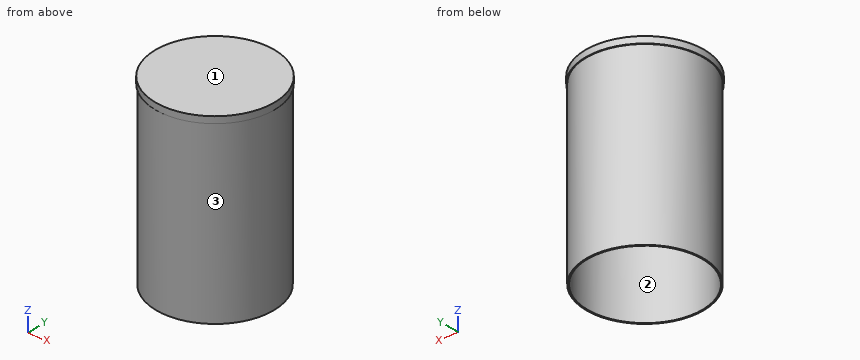
from build123d import *

# Parameters (mm, degrees)
CYLINDER_R      = 4.1
CYLINDER_DEPTH  = 3.1
SKETCH005_R     = 4.56
PAD002_DEPTH    = 0.5
SKETCH006_R     = 4.5
PAD003_DEPTH    = 13.5
SKETCH007_R     = 4.4
POCKET003_DEPTH = 13.5


with BuildPart() as part:
    # Cylinder → Cylinder (new body)
    with BuildSketch(Plane(origin=(-8, 0, 15.25), x_dir=(1, 0, 0), z_dir=(0, 0, 1))):
        Circle(CYLINDER_R)
    extrude(amount=CYLINDER_DEPTH)

    # Sketch005 → Pad002 (new body)
    with BuildSketch(Plane(origin=(-8, 0, 18.35), x_dir=(1, 0, 0), z_dir=(0, 0, 1))):
        Circle(SKETCH005_R)
    extrude(amount=PAD002_DEPTH)

    # Sketch006 → Pad003 (new body)
    with BuildSketch(Plane(origin=(-8, 0, 18.35), x_dir=(1, 0, 0), z_dir=(0, 0, -1))):
        Circle(SKETCH006_R)
    extrude(amount=PAD003_DEPTH)

    # Sketch007 → Pocket003 (cut)
    with BuildSketch(Plane(origin=(-8, 0, 4.85), x_dir=(1, 0, 0), z_dir=(0, 0, -1))):
        Circle(SKETCH007_R)
    extrude(amount=-POCKET003_DEPTH, mode=Mode.SUBTRACT)


solid = part.part
Could you check a few things on this model? Use its own coordinates, in mm. Face numbers are marked on the shaded views. Give positions to 0.01 mm unless a question says otherwise; leave off trailing zeros. Order: outer loops, then holes, each group sorted by start corner. A loop starts at its lowest first (then second) coordinate and runs counter-clockwise, first axis right, second up. Notation, with made-up numbers: (23.5, 0) -> (56.5, 0) arc R24 ccw to (56.5, 31) -> close; hole circle Ø4 at (13.5, 16). An arc over 180 degrees is marked (long way). Answer in a Markdown table with one row per item. Add a question column.
Item 1: I'm going to push flat-ended pins straight in: P1, Ø3, axis at y = -2.5, z = 8, coming from the -X side; P2, Ø2, axis at x = -4.5, z = 17, coming from the -Y side; P3, Ø2.5, axis at x = -9, y = 0, coming from the -Z side. Where does each tip first touch, or does it pass through?
Item 2: Imagine slicing it at A-A (x = -8.5). List the corners of the cut face in (y, z) for me.
Item 3: We'd pull the mould along Y, two halves only. Please class the marked faces 1, 2 and 3: pulls with the +Y half, pulls with the -Y half, needs draft (parallel to the pull), parting line crosses it, or undercut.
Item 4: Imagine slicing it at C-C (z = 11.75). List the corners of the cut face in (x, y) for me.
Item 5: Please list where these lines run through material, in increasing order: probe 1 along Z at (x, y) = (-8, -0.5); probe 2 along X at (y, z) = (-3.75, 8); probe 3 along X at (y, z) = (-4, 11).
Item 6: Imagine slicing it at B-B (y = 0). List the corners of the cut face in (x, z) for me.
Result:
| question | item | result |
|---|---|---|
| 1 | P1 | x = -12.39 |
| 1 | P2 | y = -3.74 |
| 1 | P3 | z = 18.35 |
| 2 | outline | (-4.53, 18.35) -> (-4.47, 18.35) -> (-4.47, 4.85) -> (-4.37, 4.85) -> (-4.37, 18.35) -> (4.37, 18.35) -> (4.37, 4.85) -> (4.47, 4.85) -> (4.47, 18.35) -> (4.53, 18.35) -> (4.53, 18.85) -> (-4.53, 18.85) -> close |
| 3 | face 1 | needs draft |
| 3 | face 2 | undercut |
| 3 | face 3 | parting line crosses it |
| 4 | outline | circle Ø9 at (-8, 0); hole circle Ø8.8 at (-8, 0) |
| 5 | probe 1 | 18.35 to 18.85 |
| 5 | probe 2 | -10.49 to -10.3, -5.7 to -5.51 |
| 5 | probe 3 | -10.06 to -9.83, -6.17 to -5.94 |
| 6 | outline | (-12.56, 18.35) -> (-12.5, 18.35) -> (-12.5, 4.85) -> (-12.4, 4.85) -> (-12.4, 18.35) -> (-3.6, 18.35) -> (-3.6, 4.85) -> (-3.5, 4.85) -> (-3.5, 18.35) -> (-3.44, 18.35) -> (-3.44, 18.85) -> (-12.56, 18.85) -> close |
